The model under review builds one solid part; all positions refer to its coordinate system, in mm. Face numbers are marked on the shaded views. A direction names the side the tool comes from. Round coordinates to 2 decimals unless told otherwise and drop trailing zeros. Order: outer loops, then holes, each group sorted by start corner. A loop starts at its lowest first (then second) coordinate and runs counter-clockwise, first axis right, second up. Notation, with made-up numbers: (46.25, -24) - (77.25, -24) arc R14 ccw to (77.25, -18) - close; hole circle Ø11 at (-26, 49). An arc over 180 degrees is marked (long way). One line per question, with ' | ' between items. Start each with the question number.
Item 1: Add section C-C on x = 21.5. State the section outline as (y, z) points.
Item 2: Add section A-A on y = -1.5. State the section outline as (x, z) points, and give its area (3 significant figures).
Item 3: Draft analysis for pull direction X (two halves, no side actions). For the marked faces 1, 2 and 3, state which applies: +X half, -X half, draft (parallel to the pull), parting line (faces both ways), or undercut.
Item 4: Tool access review of the marked faces 4, 5 and 6: name each direction out of +Z, -Z, +X, -X, +Y, -Y from which nothing blocks a thin tool from reaching the whole face with its end or side.
Item 5: Add section D-D on y = -16.25. State the section outline as (x, z) points, and give its area (3 significant figures).
Item 6: For L1, parallel to X at y = 0.5, z = 4; L2, parallel to Z at x = 1.5, y = -7; L3, parallel to X at y = -10.75, z = 8, list the stretches that pass through material, from the lowest coordinate up. Write a range as [from, to].
Item 7: Add section B-B on z = 22. State the section outline as (x, y) points, and give its area (3 significant figures).
Item 8: Insertion check: pin 1 Ø0.9 at (x, z) = (22, 29.5) entering from +Y; pin 2 Ø9 at (x, y) = (4.5, -5) entering from +Z. Each pin has a flat end and moves straight along its axis. Give the tip position at first contact, or say it passes through.
from build123d import *

# Parameters (mm, degrees)
F0_W     = 2
F0_H     = 10
F1_DEPTH = 40
F2_W     = 50
F2_H     = 30
F3_DEPTH = 5
F4_W     = 50
F4_H     = 30
F5_DEPTH = 5
F6_W     = 50
F6_H     = 50
F7_DEPTH = 30
F8_R     = 5
F9_R     = 5


# Not quite as in the source:
# - a feature names something its author has since deleted; it is built from what else it names


with BuildPart() as f1:
    # F0 (on Top) → F1 (new body)
    with BuildSketch(Plane.XY):
        with Locations((-24, 5)):
            Rectangle(F0_W, F0_H)
        with Locations((24, 5)):
            Rectangle(F0_W, F0_H)
        Polygon((-25, 0), (-25, -20), (25, -20), (25, 0), (23, 0), (20, 0), (20, -15), (-20, -15), (-20, 0), (-23, 0), align=None)
    extrude(amount=F1_DEPTH)

    # F2 (on face) → F3 (join)
    with BuildSketch(Plane.XY.offset(40)):
        with Locations((0, -5)):
            Rectangle(F2_W, F2_H)
    extrude(amount=F3_DEPTH)

    # F4 (on face) → F5 (join)
    with BuildSketch(Plane(origin=(0, 0, 0), x_dir=(1, 0, 0), z_dir=(0, 0, -1))):
        with Locations((0, 5)):
            Rectangle(F4_W, F4_H)
    extrude(amount=F5_DEPTH)

    # F6 (on face) → F7 (join)
    with BuildSketch(Plane(origin=(0, 10, 0), x_dir=(-1, 0, 0), z_dir=(0, 1, 0))):
        Polygon((-36, 9.5), (-36, -16), (36, -16), (36, 56), (11.5, 56), (16.5, 50.5), (-16.5, 50.5), (-11.5, 56), (-36, 56), (-36, 30.5), align=None)
        with Locations((0, 20)):
            Rectangle(F6_W, F6_H, mode=Mode.SUBTRACT)
        Polygon((-41, 4.5), (-36, 9.5), (-36, 30.5), (-41, 35.5), align=None)
    extrude(amount=-F7_DEPTH)

    # F8
    f8_edges = [f1.edges().sort_by_distance(p)[0] for p in [
        (0, 10, 0),
        (23, 10, 20),
        (0, 10, 40),
        (-23, 10, 20),
        (-36, 10, 20),
        (0, 10, -16),
    ]]
    fillet(f8_edges, radius=F8_R)

    # F9
    f9_edges = [f1.edges().sort_by_distance(p)[0] for p in [
        (20, -15, 20),
        (0, -15, 0),
        (0, -15, 40),
        (-20, -15, 20),
    ]]
    fillet(f9_edges, radius=F9_R)


solid = f1.part
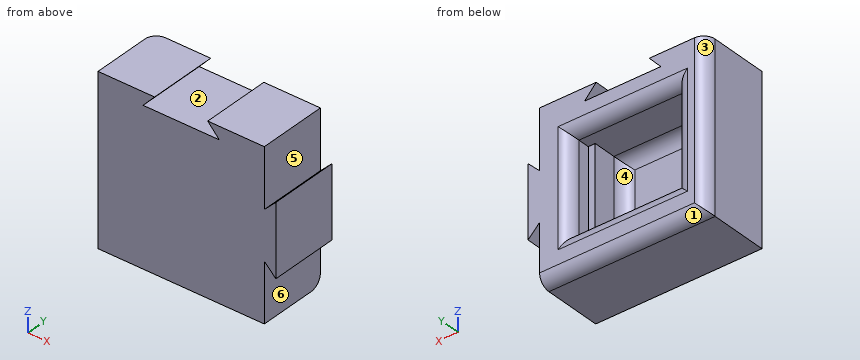
Determined:
1) outline: (-20, -16) - (5, -16) arc R5 ccw to (10, -11) - (10, -5) arc R5 ccw to (5, 0) - (0, 0) - (0, 40) - (5, 40) arc R5 ccw to (10, 45) - (10, 56) - (-20, 56) - close
2) outline: (-36, -16) - (36, -16) - (36, 9.5) - (41, 4.5) - (41, 35.5) - (36, 30.5) - (36, 56) - (11.5, 56) - (16.5, 50.5) - (-16.5, 50.5) - (-11.5, 56) - (-36, 56) - close; hole (-20, 0) - (20, 0) - (20, 40) - (-20, 40) - close | area: 3,560 mm2
3) face 1: draft | face 2: undercut | face 3: -X half
4) face 4: +Y | face 5: +Z, +Y, -Y | face 6: -Z, +Y, -Y
5) outline: (-36, -16) - (36, -16) - (36, 9.5) - (41, 4.5) - (41, 35.5) - (36, 30.5) - (36, 56) - (11.5, 56) - (16.5, 50.5) - (-16.5, 50.5) - (-11.5, 56) - (-36, 56) - close | area: 5,160 mm2
6) L1: [-36, -23], [23, 36] | L2: [-16, 0], [40, 50.5] | L3: [-36, -19.94], [19.94, 36], [37.5, 41]
7) outline: (-36, -20) - (41, -20) - (41, 10) - (28, 10) arc R5 ccw to (23, 5) - (23, 0) - (20, 0) - (20, -10) arc R5 cw to (15, -15) - (-15, -15) arc R5 cw to (-20, -10) - (-20, 0) - (-23, 0) - (-23, 5) arc R5 ccw to (-28, 10) - (-31, 10) arc R5 ccw to (-36, 5) - close | area: 1,240 mm2
8) pin 1: y = 0 | pin 2: z = 50.5
